Source: three-view drawing plus pictorial views. Frame: mm from the lowest corner of the part. A direction names the side the tool comes from. Round coordinates to 2 decimals unless told otherwise and drop trailing zeros. Order: outer loops, then holes, each group sorted by start corner. A loop starts at its lowest first (then second) coordinate and runs counter-clockwise, first axis right, second up. Notation, with made-up numbers: (41, 19.5) - (75, 19.5) arc R19 cw to (75, 42.5) - close; hole circle Ø9 at (32, -36). An arc over 180 degrees is marked (long way). Use one line per item in the form item = value. Start each with the question number.
Q1. Cut plane B-B, the plane y = 5. Return the cut outline in (x, z), and give its area (3 significant figures).
Q2. Cut plane A-A, the plane z = 1.5. Return the cut outline in (x, y), and give its area (3 significant figures).
Q3. Cut plane C-C, the plane x = 41. Return the cut outline in (y, z), and give its area (3 significant figures).
Q4. Cut plane D-D, the plane z = 19.5. Return the cut outline in (x, y) (1 decimal).
Q5. Ray query, line 1 (X direction, y = 8.25, z = 9.75); line 2 (Y direction, x = 41, z = 21.75); line 3 (Y direction, x = 5, z = 25). Return the intervals inside material, ascending. Write a range as [from, to].
Q6. Set-up query: the marked faces 1, 2 and 3. Return all of +Z, -Z, +X, -X, +Y, -Y with unobstructed straight access to the full face (end or side cutting, diameter ignored); none if empty.
Q7. Draft query along X for the marked faces 4, 5 and 6. Return one class per face: released by +X, released by -X, zero draft, split by the parting line, or undercut.
Q8. Pin query (flat end, axial travel): pin 1 Ø5 at (x, y) = (31.5, 8.5) entering from -Z; pin 2 Ø5 at (x, z) = (17, 11.5) entering from +Y (3 decimals). Return the tip coordinate at first contact, or that it passes through.
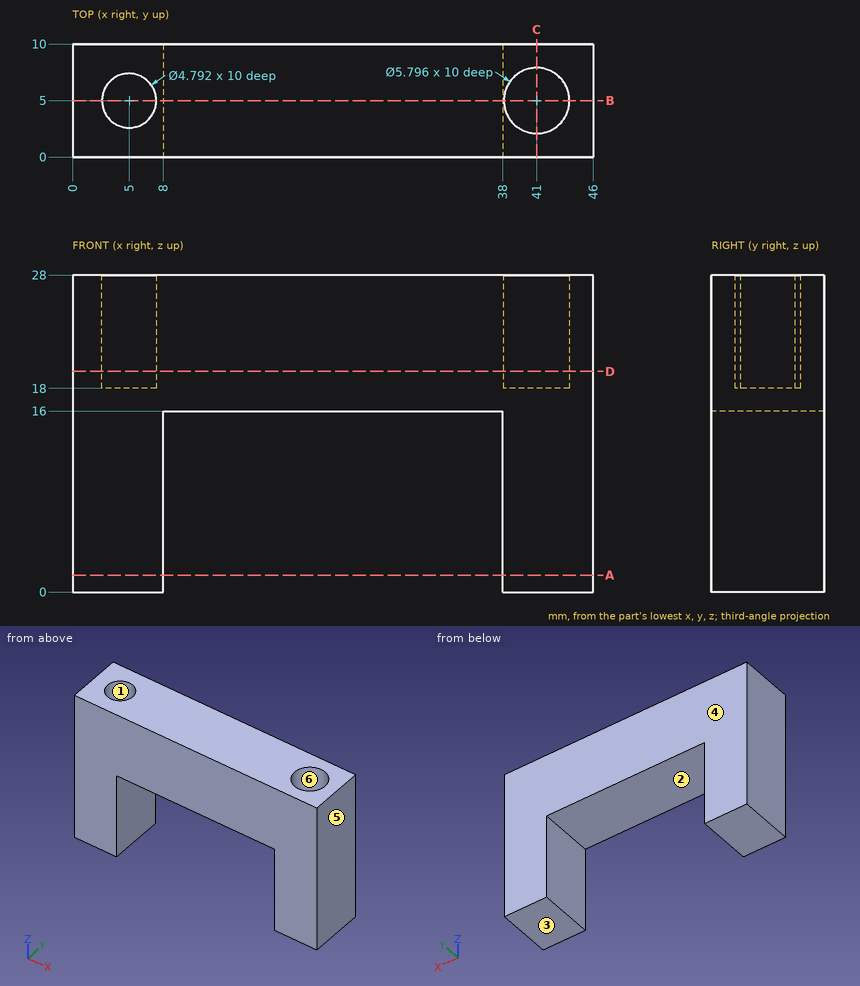
Completed:
q1.outline = (0, 0) - (8, 0) - (8, 16) - (38, 16) - (38, 0) - (46, 0) - (46, 28) - (43.9, 28) - (43.9, 18) - (38.1, 18) - (38.1, 28) - (7.4, 28) - (7.4, 18) - (2.6, 18) - (2.6, 28) - (0, 28) - close
q1.area = 702 mm2
q2.outline = (0, 0) - (8, 0) - (8, 10) - (0, 10) - close; (38, 0) - (46, 0) - (46, 10) - (38, 10) - close
q2.area = 160 mm2
q3.outline = (0, 0) - (10, 0) - (10, 28) - (7.9, 28) - (7.9, 18) - (2.1, 18) - (2.1, 28) - (0, 28) - close
q3.area = 222 mm2
q4.outline = (0, 0) - (46, 0) - (46, 10) - (0, 10) - close; hole circle Ø4.8 at (5, 5); hole circle Ø5.8 at (41, 5)
q5.line_1 = [0, 8], [38, 46]
q5.line_2 = [0, 2.1], [7.9, 10]
q5.line_3 = [0, 2.6], [7.4, 10]
q6.face_1 = +Z
q6.face_2 = -Z, +Y, -Y
q6.face_3 = -Z, +X, -X, +Y, -Y
q7.face_4 = zero draft
q7.face_5 = released by +X
q7.face_6 = undercut
q8.pin_1 = 16
q8.pin_2 = through
